Job drawing, mm, ordinate dimensions from the low corner. One solid piece. A direction names the side the tool comes from. Round coordinates to 2 decimals unless told otherwise and drop trailing zeros. Order: outer loops, then holes, each group sorted by start corner. A loop starts at its lowest first (then second) coordinate and runs counter-clockwise, first axis right, second up. Notation, with made-up numbers: (-34, -17) -> (-2, -17) arc R17 cw to (-2, 7) -> close; hole circle Ø11 at (27.25, -39). An arc over 180 degrees is marked (long way). Use CSV: the item, a comma, the result in double quotes.
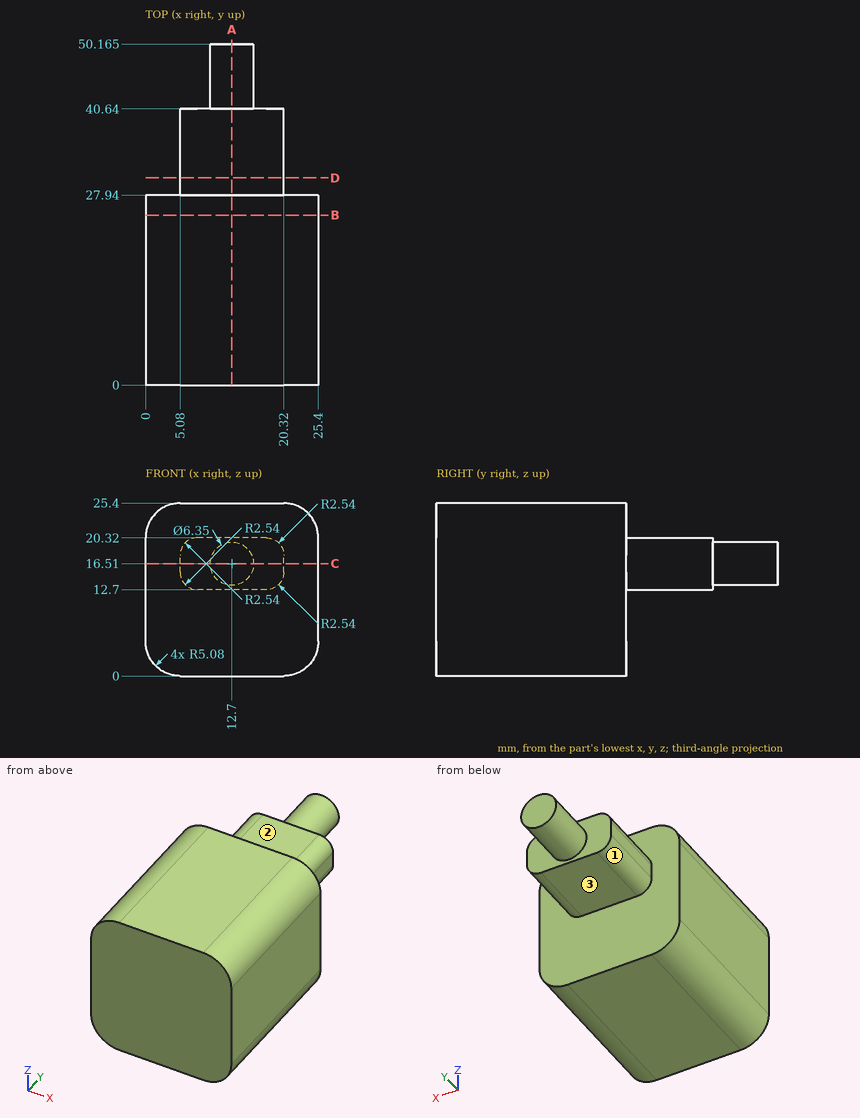
(1) Probe probe 1 along Y at (x, z) = (16.25, 9.5); probe 2 along Z at (x, y) = (15.5, 34.5); probe 3 along Z at (x, y) = (20.5, 9.5). List the from-to ranges inside material, lowest first. Write a range as [from, to].
Reply:
probe 1,"[0, 27.94]"
probe 2,"[12.7, 20.32]"
probe 3,"[0, 25.4]"
(2) Cut at C-C, the plane z = 16.51. Give the cut face in (x, y) (3 decimals), then the cut area to 3 significant figures.
Reply:
outline,"(0, 0) -> (25.4, 0) -> (25.4, 27.94) -> (20.32, 27.94) -> (20.32, 40.64) -> (15.875, 40.64) -> (15.875, 50.165) -> (9.525, 50.165) -> (9.525, 40.64) -> (5.08, 40.64) -> (5.08, 27.94) -> (0, 27.94) -> close"
area,"964 mm2"
(3) Drop flat-ended pins along their axis: P1, Ø5, axis at x = 12, y = 32.5, coming from the +Z side; P2, Ø11, axis at x = 11.5, y = 35, coming from the -Z side; P3, Ø2, axis at y = 32, z = 16.5, coming from the -X side. Give the stop position or say it passes through.
Reply:
P1,"z = 20.32"
P2,"z = 12.7"
P3,"x = 5.08"
(4) Cut at A-A, the plane x = 12.7. Give the cut face in (y, z) (3 decimals).
Reply:
outline,"(0, 0) -> (27.94, 0) -> (27.94, 12.7) -> (40.64, 12.7) -> (40.64, 13.335) -> (50.165, 13.335) -> (50.165, 19.685) -> (40.64, 19.685) -> (40.64, 20.32) -> (27.94, 20.32) -> (27.94, 25.4) -> (0, 25.4) -> close"
(5) Cut at D-D, the plane y = 30.5. Give the cut face in (x, z).
Reply:
outline,"(5.08, 15.24) arc R2.54 ccw to (7.62, 12.7) -> (17.78, 12.7) arc R2.54 ccw to (20.32, 15.24) -> (20.32, 17.78) arc R2.54 ccw to (17.78, 20.32) -> (7.62, 20.32) arc R2.54 ccw to (5.08, 17.78) -> close"
(6) Which spindle directions (+Z, -Z, +X, -X, +Y, -Y) get a long thin tool onto all of the face, cutting with end or side? Do the marked faces 1, 2 and 3. Say none if no direction does.
Reply:
face 1,"-Z, -X, +Y"
face 2,"+Z, +X, -X, +Y"
face 3,"-Z, +X, -X, +Y"
(7) Cut at B-B, the plane y = 25. Give the cut face in (x, z).
Reply:
outline,"(0, 5.08) arc R5.08 ccw to (5.08, 0) -> (20.32, 0) arc R5.08 ccw to (25.4, 5.08) -> (25.4, 20.32) arc R5.08 ccw to (20.32, 25.4) -> (5.08, 25.4) arc R5.08 ccw to (0, 20.32) -> close"
